Model file for the job. Use its own axes, mm. Coordinates: 2 decimals unless noted, no trailing zeros. Write each loop counter-clockwise with the first axis right and the second up, starting at its lowest first coordinate (ties: lowest second). Pieces come first, ordered by that corner, then holes. Notation, with made-up numbers: M 81,69 L 113,69 A18 cw 113,83 Z; hole C 46,66 d7. An arc over 180 degrees is marked long. Answer in a Markdown table with one row per item. Add a question column.
```python
from build123d import *

# Parameters (mm, degrees)
SKETCH_W     = 50.75
SKETCH_H     = 25
PAD_DEPTH    = 1.6
FILLET_R     = 2
SKETCH001_R  = 1.3
POCKET_DEPTH = 1.601


with BuildPart() as part:
    # Sketch → Pad (new body)
    with BuildSketch(Plane.XZ):
        Rectangle(SKETCH_W, SKETCH_H)
    extrude(amount=-PAD_DEPTH)

    # Fillet
    fillet_edges = [part.edges().sort_by_distance(p)[0] for p in [
        (25.375, 0.8, 12.5),
        (-25.375, 0.8, 12.5),
        (-25.375, 0.8, -12.5),
        (25.375, 0.8, -12.5),
    ]]
    fillet(fillet_edges, radius=FILLET_R)

    # Sketch001 → Pocket (cut, through all)
    with BuildSketch(Plane.XZ):
        with Locations((-22.625, 0)):
            Circle(SKETCH001_R)
        with Locations((7.125, 10.25)):
            Circle(SKETCH001_R)
        with Locations((7.125, -10.25)):
            Circle(SKETCH001_R)
    extrude(amount=-POCKET_DEPTH, mode=Mode.SUBTRACT)


solid = part.part
```
1) Flat gauge pin, fed straight in: pin 1 Ø2 at (x, z) = (-22.625, 0) entering from -Y. Where does the tip first touch, or does it go through?
2) Slice it at D-D (x = -22). Give the cut face in (y, z), then the cut area to 3 significant figures.
3) Drill centre lines: probe 1 along Z at (x, y) = (6, 0.9); probe 2 along Z at (x, y) = (6.5, 1.1); probe 3 along X at (y, z) = (1.35, 1) (3 decimals). Where is each one in solid material? Low to high.
4) Slice it at C-C (x = 7). Give the cut face in (y, z), then the cut area to 3 significant figures.
5) Slice it at A-A (z = 0). Give the cut face in (x, y) (3 decimals), then the cut area to 3 significant figures.
6) Two-plate mould, pull along X, no slides. Class faces 1 (the face through (7.82, 0.79, 11.35)), 2 (the face through (8.365, 0.789, -9.86)), 3 (the face through (0, 0, 0)), 4 (the face through (-25.375, 1, 0)): released by +X, released by -X, zero draft, split by the parting line, or undercut.
7) Slice it at B-B (y = 1.3). Give the cut face in (x, z) (3 decimals).
Ans:
| question | item | result |
|---|---|---|
| 1 | pin 1 | passes through |
| 2 | outline | M 0,-12.5 L 1.6,-12.5 L 1.6,-1.14 L 0,-1.14 Z; M 0,1.14 L 1.6,1.14 L 1.6,12.5 L 0,12.5 Z |
| 2 | area | 36.4 mm2 |
| 3 | probe 1 | z = -12.5 to -10.9, -9.6 to 9.6, 10.9 to 12.5 |
| 3 | probe 2 | z = -12.5 to -11.39, -9.11 to 9.11, 11.39 to 12.5 |
| 3 | probe 3 | x = -25.375 to -23.456, -21.794 to 25.375 |
| 4 | outline | M 0,-12.5 L 1.6,-12.5 L 1.6,-11.54 L 0,-11.54 Z; M 0,-8.96 L 1.6,-8.96 L 1.6,8.96 L 0,8.96 Z; M 0,11.54 L 1.6,11.54 L 1.6,12.5 L 0,12.5 Z |
| 4 | area | 31.7 mm2 |
| 5 | outline | M -25.375,0 L -23.925,0 L -23.925,1.6 L -25.375,1.6 Z; M -21.325,0 L 25.375,0 L 25.375,1.6 L -21.325,1.6 Z |
| 5 | area | 77.0 mm2 |
| 6 | face 1 | undercut |
| 6 | face 2 | undercut |
| 6 | face 3 | zero draft |
| 6 | face 4 | released by -X |
| 7 | outline | M -25.375,-10.5 A2 ccw -23.375,-12.5 L 23.375,-12.5 A2 ccw 25.375,-10.5 L 25.375,10.5 A2 ccw 23.375,12.5 L -23.375,12.5 A2 ccw -25.375,10.5 Z; hole C -22.625,0 d2.6; hole C 7.125,-10.25 d2.6; hole C 7.125,10.25 d2.6 |
